```python
from build123d import *

# Parameters (mm, degrees)
BOSS_EXTRUDE1_DEPTH = 12.7


with BuildPart() as part:
    # Sketch1 → Boss-Extrude1 (new body)
    with BuildSketch(Plane(origin=(0, 0, 0), x_dir=(0, -1, 0), z_dir=(-1, 0, 0))):
        with BuildLine():
            ThreePointArc((-8.177440487, -6.029516323), (-7.943407862, -6.334656387), (-7.697995454, -6.630721377))
            ThreePointArc((-7.697995454, -6.630721377), (-6.273562142, -6.180849316), (-5.15957287, -5.185649317))
            ThreePointArc((-5.15957287, -5.185649317), (-4.560952599, -5.719253661), (-3.907521288, -6.184127135))
            ThreePointArc((-3.907521288, -6.184127135), (-4.629883612, -7.491639203), (-4.75151021, -8.98046495))
            ThreePointArc((-4.75151021, -8.98046495), (-4.408258789, -9.153843698), (-4.058692066, -9.314108584))
            ThreePointArc((-4.058692066, -9.314108584), (-2.970514168, -8.29074941), (-2.398645612, -6.910763363))
            ThreePointArc((-2.398645612, -6.910763363), (-1.627785136, -7.131792663), (-0.837362826, -7.267115971))
            ThreePointArc((-0.837362826, -7.267115971), (-0.920880567, -8.758564905), (-0.384485064, -10.152722356))
            ThreePointArc((-0.384485064, -10.152722356), (0, -10.16), (0.384485064, -10.152722356))
            ThreePointArc((0.384485064, -10.152722356), (0.920880567, -8.758564905), (0.837362826, -7.267115971))
            ThreePointArc((0.837362826, -7.267115971), (1.627785136, -7.131792663), (2.398645612, -6.910763363))
            ThreePointArc((2.398645612, -6.910763363), (2.970514168, -8.29074941), (4.058692066, -9.314108584))
            ThreePointArc((4.058692066, -9.314108584), (4.408258789, -9.153843698), (4.75151021, -8.98046495))
            ThreePointArc((4.75151021, -8.98046495), (4.629883612, -7.491639203), (3.907521288, -6.184127135))
            ThreePointArc((3.907521288, -6.184127135), (4.560952599, -5.719253661), (5.15957287, -5.185649317))
            ThreePointArc((5.15957287, -5.185649317), (6.273562142, -6.180849316), (7.697995454, -6.630721377))
            ThreePointArc((7.697995454, -6.630721377), (7.943407862, -6.334656387), (8.177440487, -6.029516323))
            ThreePointArc((8.177440487, -6.029516323), (7.421881426, -4.740902478), (6.203747236, -3.876296077))
            ThreePointArc((6.203747236, -3.876296077), (6.590767462, -3.173946328), (6.898583443, -2.433453825))
            ThreePointArc((6.898583443, -2.433453825), (8.334054192, -2.846756211), (9.812616434, -2.634038481))
            ThreePointArc((9.812616434, -2.634038481), (9.905267588, -2.260812689), (9.983728385, -1.884348041))
            ThreePointArc((9.983728385, -1.884348041), (8.7438846, -1.051171874), (7.271244959, -0.800717041))
            ThreePointArc((7.271244959, -0.800717041), (7.3152, 0), (7.271244959, 0.800717041))
            ThreePointArc((7.271244959, 0.800717041), (8.7438846, 1.051171874), (9.983728385, 1.884348041))
            ThreePointArc((9.983728385, 1.884348041), (9.905267588, 2.260812689), (9.812616434, 2.634038481))
            ThreePointArc((9.812616434, 2.634038481), (8.334054192, 2.846756211), (6.898583443, 2.433453825))
            ThreePointArc((6.898583443, 2.433453825), (6.590767462, 3.173946328), (6.203747236, 3.876296077))
            ThreePointArc((6.203747236, 3.876296077), (7.421881426, 4.740902478), (8.177440487, 6.029516323))
            ThreePointArc((8.177440487, 6.029516323), (7.943407862, 6.334656387), (7.697995454, 6.630721377))
            ThreePointArc((7.697995454, 6.630721377), (6.273562142, 6.180849316), (5.15957287, 5.185649317))
            ThreePointArc((5.15957287, 5.185649317), (4.560952599, 5.719253661), (3.907521288, 6.184127135))
            ThreePointArc((3.907521288, 6.184127135), (4.629883612, 7.491639203), (4.75151021, 8.98046495))
            ThreePointArc((4.75151021, 8.98046495), (4.408258789, 9.153843698), (4.058692066, 9.314108584))
            ThreePointArc((4.058692066, 9.314108584), (2.970514168, 8.29074941), (2.398645612, 6.910763363))
            ThreePointArc((2.398645612, 6.910763363), (1.627785136, 7.131792663), (0.837362826, 7.267115971))
            ThreePointArc((0.837362826, 7.267115971), (0.920880567, 8.758564905), (0.384485064, 10.152722356))
            ThreePointArc((0.384485064, 10.152722356), (0, 10.16), (-0.384485064, 10.152722356))
            ThreePointArc((-0.384485064, 10.152722356), (-0.920880567, 8.758564905), (-0.837362826, 7.267115971))
            ThreePointArc((-0.837362826, 7.267115971), (-1.627785136, 7.131792663), (-2.398645612, 6.910763363))
            ThreePointArc((-2.398645612, 6.910763363), (-2.970514168, 8.29074941), (-4.058692066, 9.314108584))
            ThreePointArc((-4.058692066, 9.314108584), (-4.408258789, 9.153843698), (-4.75151021, 8.98046495))
            ThreePointArc((-4.75151021, 8.98046495), (-4.629883612, 7.491639203), (-3.907521288, 6.184127135))
            ThreePointArc((-3.907521288, 6.184127135), (-4.560952599, 5.719253661), (-5.15957287, 5.185649317))
            ThreePointArc((-5.15957287, 5.185649317), (-6.273562142, 6.180849316), (-7.697995454, 6.630721377))
            ThreePointArc((-7.697995454, 6.630721377), (-7.943407862, 6.334656387), (-8.177440487, 6.029516323))
            ThreePointArc((-8.177440487, 6.029516323), (-7.421881426, 4.740902478), (-6.203747236, 3.876296077))
            ThreePointArc((-6.203747236, 3.876296077), (-6.590767462, 3.173946328), (-6.898583443, 2.433453825))
            ThreePointArc((-6.898583443, 2.433453825), (-8.334054192, 2.846756211), (-9.812616434, 2.634038481))
            ThreePointArc((-9.812616434, 2.634038481), (-9.905267588, 2.260812689), (-9.983728385, 1.884348041))
            ThreePointArc((-9.983728385, 1.884348041), (-8.7438846, 1.051171874), (-7.271244959, 0.800717041))
            ThreePointArc((-7.271244959, 0.800717041), (-7.3152, 0), (-7.271244959, -0.800717041))
            ThreePointArc((-7.271244959, -0.800717041), (-8.7438846, -1.051171874), (-9.983728385, -1.884348041))
            ThreePointArc((-9.983728385, -1.884348041), (-9.905267588, -2.260812689), (-9.812616434, -2.634038481))
            ThreePointArc((-9.812616434, -2.634038481), (-8.334054192, -2.846756211), (-6.898583443, -2.433453825))
            ThreePointArc((-6.898583443, -2.433453825), (-6.590767462, -3.173946328), (-6.203747236, -3.876296077))
            ThreePointArc((-6.203747236, -3.876296077), (-7.421881426, -4.740902478), (-8.177440487, -6.029516323))
        make_face()
        with BuildLine():
            Line((-5.1054, 1), (-3.872983346, 1))
            ThreePointArc((-3.872983346, 1), (4, 0), (-3.872983346, -1))
            Line((-3.872983346, -1), (-5.1054, -1))
            Line((-5.1054, -1), (-5.1054, 1))
        make_face(mode=Mode.SUBTRACT)
    extrude(amount=-BOSS_EXTRUDE1_DEPTH)


solid = part.part
```
Part model, mm, in its own coordinate system. Round coordinates to 2 decimals unless told otherwise and drop trailing zeros. Loops run counter-clockwise (first coordinate to the right, second up) from the corner with the lowest first, then second, coordinate; pieces in that order, holes last. Notation, with made-up numbers: (-40, -31) -> (-15, -31) arc R27 cw to (-15, 3) -> close; hole circle Ø10 at (79, 79.25). An arc over 180 degrees is marked (long way). Use CSV: the item, a comma, the result in double quotes. Start each with the question number.
1) Wall check: L1, parallel to Z at x = 5.25, y = 0; L2, parallel to Z at x = 3.75, y = -8; L3, parallel to Y at x = 6.5, z = 9.25. Give the ranges that are in metal, low to high. Write a range as [from, to].
2) Cut at A-A, the plane y = 0. Write the cut outline in (x, z), plus the area to 3 significant figures.
3) Cut at B-B, the plane z = 0. Write the cut outline in (x, y), plus the area to 3 significant figures.
4) Drop flat-ended pins along their axis: P1, Ø2, axis at x = 11, z = -7.5, coming from the -Y side; P2, Ø4, axis at x = 8, y = -7.5, coming from the -Z side; P3, Ø1.6, axis at x = 9.5, z = -0.5, coming from the -Y side. Give the stop position or say it passes through.
Determined:
1,L1,"z = [-10.16, -4], [4, 10.16]"
1,L2,"z = [-6.26, -5.59], [-2.81, -0.84], [0.84, 2.81], [5.59, 6.26]"
1,L3,"y = [-4.2, -3.96], [-0.81, 0.81], [3.96, 4.2]"
2,outline,"(0, -10.16) -> (12.7, -10.16) -> (12.7, -4) -> (0, -4) -> close; (0, 4) -> (12.7, 4) -> (12.7, 10.16) -> (0, 10.16) -> close"
2,area,"156 mm2"
3,outline,"(0, -7.32) -> (12.7, -7.32) -> (12.7, -4) -> (0, -4) -> close; (0, 5.11) -> (12.7, 5.11) -> (12.7, 7.32) -> (0, 7.32) -> close"
3,area,"70.2 mm2"
4,P1,"stops at y = -7.81"
4,P2,"stops at z = -6.63"
4,P3,"stops at y = -9.25"
